Can you work these out from the model? Positions are in its coordinate system, mm. Face numbers are marked on the shaded views. Give positions to 0.01 mm unless a question says otherwise; leave off trailing zeros. Order: outer loops, then holes, each group sorted by start corner. A loop starts at its lowest first (then second) coordinate and runs counter-clockwise, first axis right, second up. Notation, with made-up numbers: M -35,-4 L -27,-4 A19 ccw -27,16 Z; hole C 19,-1.75 d5. An arc over 180 degrees is marked long. Write each question's results on one line, items separated by ' | '.
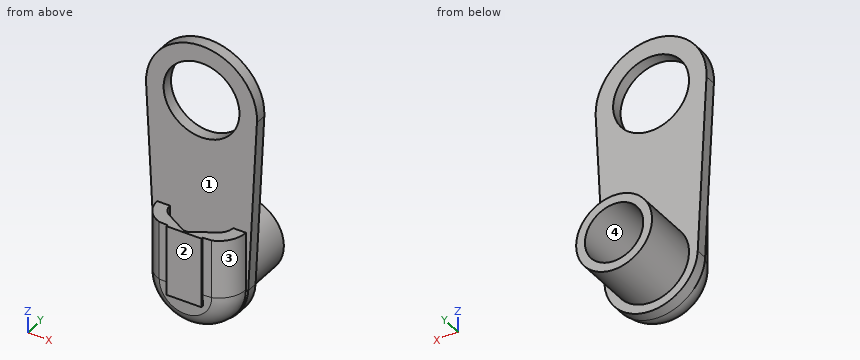
Autodesk Inventor part; units mm, degrees
ref_plane "Arbeitsebene1" through (0, 0, -190) normal (-1, 0, 0) x (0, -1, 0)
ref_plane "YZ Plane" through (0, 0, 0) normal (1, 0, 0) x (0, 1, 0)
ref_plane "XZ Plane" through (0, 0, 0) normal (0, 1, 0) x (-1, 0, 0)
sketch "Skizze1" plane through (0, 0, 0) normal (0, 1, 0) x (-1, 0, 0)
  circle A0 centre (0, 0) radius 32.5
  circle A1 centre (0, 0) radius 47.5
  line L0 (0, 0) -> (0, -150) construction
  circle A2 centre (0, -150) radius 25
  circle A3 centre (0, -150) radius 40
  line L1 (47.4406, -2.375) -> (39.95, -152)
  line L2 (-47.4406, -2.375) -> (-39.95, -152)
  dimension "d0" = 65
  dimension "d1" = 15
  dimension "d2" = 150
  dimension "d3" = 50
  dimension "d4" = 15
extrude "Extrusion1" add sketch "Skizze1" along normal blind 10
sketch "Skizze2" plane through (0, 10, 0) normal (0, 1, 0) x (1, 0, 0)
  circle A0 centre (0, 150) radius 25
  circle A1 centre (0, 150) radius 32.5
  point P0 (0, 0)
  dimension "d7" = 7.5
extrude "Extrusion2" add sketch "Skizze2" along normal blind 50
ref_plane "Arbeitsebene1" through (0, 0, -190) normal (-1, 0, 0) x (0, -1, 0)
sketch "Skizze3" plane through (0, 0, -190) normal (-1, 0, 0) x (0, -1, 0)
  line L0 (0, 38) -> (0, 0)
  line L1 (0, 10.9925) -> (10.9925, 10.9925) construction
  line L2 (0, 10.9925) -> (0, 0) construction
  line L3 (0, 0) -> (0, 3)
  line L4 (0, 38) -> (-10, 38) construction
  line L5 (0, 38) -> (16.612, 38) construction
  arc A0 (0, 10.9925) -> (10.4174, 17.007) centre (0, 23.0214) ccw
  line L6 (0, 23.0214) -> (12.0289, 23.0214) construction
  line L7 (0, 23.0214) -> (0, 10.9925) construction
  line L8 (-10.9478, 2.8205) -> (-10.9478, 33.9693) construction
  line L9 (-10.9478, 33.9693) -> (20.2009, 33.9693) construction
  line L10 (22.6543, 38) -> (21.7274, 15.548)
  arc A1 (0, 0.0447) -> (21.7274, 15.548) centre (0, 23.0214) ccw
  line L11 (0, 10.9925) -> (0, 3)
  line L12 (10.4174, 17.007) -> (22.6543, 38)
  point P0 (0, 190)
  dimension "d12" = 90
revolve "Umdrehung1" add sketch "Skizze3" angle 180 mid plane about axis through (0, 0, -152) along (0, -1, 0)
sketch "Skizze4" plane through (-37.9553, 0, -152) normal (0, 0, 1) x (1, 0, 0)
  line L0 (64.9628, 0) -> (75.9106, 0)
  arc A0 (58.9484, -10.4174) -> (64.9628, 0) centre (52.9339, 0) ccw
  line L1 (58.9484, -10.4174) -> (37.9553, -22.6543)
  line L2 (37.9553, -22.6543) -> (60.4073, -21.7274)
  arc A1 (60.4073, -21.7274) -> (75.9106, 0) centre (52.9339, 0) ccw
  line L3 (0, 0) -> (10.9478, 0)
  arc A2 (0, 0) -> (15.5034, -21.7274) centre (22.9768, 0) ccw
  line L4 (15.5034, -21.7274) -> (37.9553, -22.6543)
  line L5 (37.9553, -22.6543) -> (16.9623, -10.4174)
  arc A3 (10.9478, 0) -> (16.9623, -10.4174) centre (22.9768, 0) ccw
  point P0 (37.9553, 0)
extrude "Extrusion3" add sketch "Skizze4" along normal blind 50
sketch "Skizze5" plane through (-37.9553, 0, -102) normal (0, 0, 1) x (1, 0, 0)
  line L0 (22.9553, -21.6543) -> (52.9553, -21.6543)
  line L1 (52.9553, -21.6543) -> (52.9553, -23.6543)
  line L2 (52.9553, -23.6543) -> (22.9553, -23.6543)
  line L3 (22.9553, -23.6543) -> (22.9553, -21.6543)
  line L4 (37.9553, -22.6543) -> (16.9623, -10.4174)
  line L5 (22.9553, -21.6543) -> (52.9553, -23.6543) construction
  line L6 (52.9553, -21.6543) -> (22.9553, -23.6543) construction
  point P0 (37.9553, 0)
  dimension "d16" = 30
  dimension "d17" = 2
extrude "Extrusion4" add sketch "Skizze5" against normal blind 60
properties part number "Absaugschuh" material "PET-Kunststoff"
(1) Imagine slicing it at C-C, the plane z = -76. Write out the boundary of the cut face in (x, y), plus the area to 3 significant figures.
Data:
outline: M -43.75,0 L 43.75,0 L 43.75,10 L -43.75,10 Z | area: 875 mm2
(2) Imagine slicing it at B-B, the plane y = 43.5. Write out the boundary of the cut face in (x, z).
Data:
outline: C 0,-150 d65; hole C 0,-150 d50
(3) Will these pins go through, and if not, where does the flat tip stop? P1, Ø1, axis at x = 31, z = -119, coming from the +Y side; P2, Ø7, axis at x = 5.5, y = -7.5, coming from the +Z side; P3, Ø0.5, axis at x = 4.5, y = -23, coming from the -Z side.
Data:
P1: stops at y = 10 | P2: stops at z = -171.13 | P3: stops at z = -162
(4) I need wall thicknesses on L1, parallel to Z at x = 0, y = 41; L2, parallel to X at y = 22.5, z = -150; L3, parallel to Y at x = -15, z = -49. Which ranges of each line are inside material? Lowest first, please. Write a range as from..to.
Data:
L1: z = -182.5..-175, -125..-117.5 | L2: x = -32.5..-25, 25..32.5 | L3: y = 0..10
(5) We'd pull the mould along X, two halves only. Please class the marked faces 1, 2, 3 and 4: +X half, -X half, draft (parallel to the pull), parting line (faces both ways), or undercut.
Data:
face 1: undercut | face 2: draft | face 3: +X half | face 4: undercut
(6) Imagine slicing it at A-A, the plane z = 0. Write out the boundary of the cut face in (x, y).
Data:
outline: M -47.5,0 L -32.5,0 L -32.5,10 L -47.5,10 Z; M 32.5,0 L 47.5,0 L 47.5,10 L 32.5,10 Z
